```python
from build123d import *

# Parameters (mm, degrees)
SKETCH_1_W          = 95
SKETCH_1_H          = 45
EXTRUDE_1_DEPTH     = 19.3
SHELL_1_T           = -4
FILLET_1_R          = 4.5
SKETCH_2_W          = 71.05
SKETCH_2_H          = 22.55
CUT_EXTRUDE_1_DEPTH = 4.5
EXTRUDE_3_DEPTH     = 6
SKETCH_7_R          = 1.55
CUT_EXTRUDE_2_DEPTH = 4
SKETCH_8_R          = 0.75
EXTRUDE_5_DEPTH     = 5
EXTRUDE_6_DEPTH     = 2.5
SKETCH_9_W          = 1.5
SKETCH_9_H          = 22.55
EXTRUDE_7_DEPTH     = 2.5
SKETCH_10_W         = 74.05
SKETCH_10_H         = 26.962586992
CUT_EXTRUDE_3_DEPTH = 9
SKETCH_12_W         = 4.67
SKETCH_12_H         = 2.36
CUT_EXTRUDE_4_DEPTH = 24
FILLET_2_R          = 1
FILLET_3_R          = 1


with BuildPart() as part:
    # Sketch 1 → Extrude 1 (new body)
    with BuildSketch(Plane(origin=(0, 0, 0), x_dir=(1, 0, 0), z_dir=(0, 1, 0))):
        with Locations((47.5, -22.5)):
            Rectangle(SKETCH_1_W, SKETCH_1_H)
    extrude(amount=EXTRUDE_1_DEPTH)

    # Shell 1
    shell_1_openings = [part.faces().sort_by_distance(p)[0] for p in [
        (47.5, 19.3, 22.5),
    ]]
    offset(amount=SHELL_1_T, openings=shell_1_openings, kind=Kind.INTERSECTION)

    # Fillet 1
    fillet_1_edges = [part.edges().sort_by_distance(p)[0] for p in [
        (47.5, 0, 0),
        (95, 0, 22.5),
        (47.5, 0, 45),
        (0, 0, 22.5),
        (0, 9.65, 0),
        (95, 9.65, 0),
        (95, 9.65, 45),
        (0, 9.65, 45),
    ]]
    fillet(fillet_1_edges, radius=FILLET_1_R)

    # Sketch 2 → Cut-Extrude 1 (cut)
    with BuildSketch(Plane(origin=(0, 0, 0), x_dir=(-1, 0, 0), z_dir=(0, -1, 0))):
        with Locations((-47.5, -22.5)):
            Rectangle(SKETCH_2_W, SKETCH_2_H)
    extrude(amount=-CUT_EXTRUDE_1_DEPTH, mode=Mode.SUBTRACT)

    # Sketch 6 → Extrude 3 (add)
    with BuildSketch(Plane(origin=(0, 4, 0), x_dir=(1, 0, 0), z_dir=(0, 1, 0))):
        Polygon((11.975, -11.225), (11.975, -13.725), (7.475, -13.725), (7.475, -5.725), (15.475, -5.725), (15.475, -11.225), align=None)
        Polygon((11.975, -33.775), (11.975, -31.775), (7.475, -31.775), (7.475, -40.725), (15.475, -40.725), (15.475, -33.775), align=None)
        Polygon((87.525, -40.725), (79.525, -40.725), (79.525, -33.775), (83.025, -33.775), (83.025, -31.775), (87.525, -31.775), align=None)
        Polygon((79.525, -5.725), (79.525, -11.225), (83.025, -11.225), (83.025, -13.725), (87.525, -13.725), (87.525, -5.725), align=None)
    extrude(amount=EXTRUDE_3_DEPTH)

    # Sketch 7 → Cut-Extrude 2 (cut)
    with BuildSketch(Plane(origin=(0, 10, 0), x_dir=(1, 0, 0), z_dir=(0, 1, 0))):
        with Locations(Location((9.975, -7.725, 0), (0, 0, 270))):
            Circle(SKETCH_7_R)
        with Locations(Location((85.025, -7.725, 0), (0, 0, 90))):
            Circle(SKETCH_7_R)
        with Locations(Location((9.975, -38.725, 0), (0, 0, 270))):
            Circle(SKETCH_7_R)
        with Locations(Location((85.025, -38.725, 0), (0, 0, 90))):
            Circle(SKETCH_7_R)
    extrude(amount=-CUT_EXTRUDE_2_DEPTH, mode=Mode.SUBTRACT)

    # Sketch 8 → Extrude 5 (add)
    with BuildSketch(Plane(origin=(0, 19.3, 0), x_dir=(1, 0, 0), z_dir=(0, 1, 0))):
        with Locations((6, -43)):
            Circle(SKETCH_8_R)
        with Locations((6, -2)):
            Circle(SKETCH_8_R)
        with Locations((89, -2)):
            Circle(SKETCH_8_R)
        with BuildLine():
            ThreePointArc((89.75, -2), (89.530330086, -2.530330086), (89, -2.75))
            Line((89, -2.75), (92.25, -2.75))
            Line((92.25, -2.75), (92.25, -6))
            ThreePointArc((92.25, -6), (92.469669914, -5.469669914), (93, -5.25))
            Line((93, -5.25), (93, -2))
            Line((93, -2), (89.75, -2))
        make_face()
        with Locations((93, -6)):
            Circle(SKETCH_8_R)
        with Locations((93, -39)):
            Circle(SKETCH_8_R)
        with BuildLine():
            Line((92.25, -42.25), (89, -42.25))
            ThreePointArc((89, -42.25), (89.530330086, -42.469669914), (89.75, -43))
            Line((89.75, -43), (93, -43))
            Line((93, -43), (93, -39.75))
            ThreePointArc((93, -39.75), (92.469669914, -39.530330086), (92.25, -39))
            Line((92.25, -39), (92.25, -42.25))
        make_face()
        with Locations((89, -43)):
            Circle(SKETCH_8_R)
        with BuildLine():
            Line((6, -42.25), (2.75, -42.25))
            Line((2.75, -42.25), (2.75, -43))
            Line((2.75, -43), (5.25, -43))
            ThreePointArc((5.25, -43), (5.469669914, -42.469669914), (6, -42.25))
        make_face()
        with BuildLine():
            Line((5.25, -2), (2.75, -2))
            Line((2.75, -2), (2.75, -2.75))
            Line((2.75, -2.75), (6, -2.75))
            ThreePointArc((6, -2.75), (5.469669914, -2.530330086), (5.25, -2))
        make_face()
    extrude(amount=EXTRUDE_5_DEPTH)

    # Sketch 8_4 → Extrude 6 (add)
    with BuildSketch(Plane(origin=(0, 19.3, 0), x_dir=(1, 0, 0), z_dir=(0, 1, 0))):
        with BuildLine():
            ThreePointArc((6.75, -2), (6.530330086, -2.530330086), (6, -2.75))
            Line((6, -2.75), (89, -2.75))
            ThreePointArc((89, -2.75), (88.469669914, -2.530330086), (88.25, -2))
            Line((88.25, -2), (6.75, -2))
        make_face()
        with BuildLine():
            ThreePointArc((93, -6.75), (92.469669914, -6.530330086), (92.25, -6))
            Line((92.25, -6), (92.25, -39))
            ThreePointArc((92.25, -39), (92.469669914, -38.469669914), (93, -38.25))
            Line((93, -38.25), (93, -6.75))
        make_face()
        with BuildLine():
            Line((89, -42.25), (6, -42.25))
            ThreePointArc((6, -42.25), (6.530330086, -42.469669914), (6.75, -43))
            Line((6.75, -43), (88.25, -43))
            ThreePointArc((88.25, -43), (88.469669914, -42.469669914), (89, -42.25))
        make_face()
    extrude(amount=EXTRUDE_6_DEPTH)

    # Sketch 9 → Extrude 7 (add)
    with BuildSketch(Plane(origin=(0, 19.3, 0), x_dir=(1, 0, 0), z_dir=(0, 1, 0))):
        with Locations((2.75, -22.5)):
            Rectangle(SKETCH_9_W, SKETCH_9_H)
    extrude(amount=EXTRUDE_7_DEPTH)

    # Sketch 10 → Cut-Extrude 3 (cut)
    with BuildSketch(Plane(origin=(0, 10, 0), x_dir=(1, 0, 0), z_dir=(0, 1, 0))):
        with Locations((47.5, -23.243706504)):
            Rectangle(SKETCH_10_W, SKETCH_10_H)
    extrude(amount=-CUT_EXTRUDE_3_DEPTH, mode=Mode.SUBTRACT)

    # Sketch 12 → Cut-Extrude 4 (cut)
    with BuildSketch(Plane(origin=(95, 0, 0), x_dir=(0, 0, -1), z_dir=(1, 0, 0))):
        with Locations((-24.835, 18.12)):
            Rectangle(SKETCH_12_W, SKETCH_12_H)
        with Locations((-20.165, 18.12)):
            Rectangle(SKETCH_12_W, SKETCH_12_H)
        Polygon((-27.17, 19.3), (-22.5, 19.3), (-17.83, 19.3), (-17.83, 20.8), (-27.17, 20.8), align=None)
    extrude(amount=-CUT_EXTRUDE_4_DEPTH, mode=Mode.SUBTRACT)

    # Fillet 2
    fillet_2_edges = [part.edges().sort_by_distance(p)[0] for p in [
        (93, 16.94, 27.17),
    ]]
    fillet(fillet_2_edges, radius=FILLET_2_R)

    # Fillet 3
    fillet_3_edges = [part.edges().sort_by_distance(p)[0] for p in [
        (93, 16.94, 17.83),
    ]]
    fillet(fillet_3_edges, radius=FILLET_3_R)


solid = part.part
```
Check sheet for the modelled part. Datum: model origin and axes. Units: mm. A direction names the side the tool comes from. Round coordinates to 2 decimals unless told otherwise and drop trailing zeros. Loops run counter-clockwise (first coordinate to the right, second up) from the corner with the lowest first, then second, coordinate; pieces in that order, holes last. Notation, with made-up numbers: (-9.5, -17.75) - (26.5, -17.75) arc R31 ccw to (26.5, 15.25) - close; hole circle Ø9 at (11.5, -15.5). An arc over 180 degrees is marked (long way). Answer as a JSON object with one key per item and string values. Group by question number.
Q1. Sectioned sample at A-A, the plane z = 21.5. Enter the section's corners in (x, y) (3 decimals), plus the area to 3 significant figures.
Q2. Set-up check for faces 1 (the face through (91, 12, 23)), 2 (the face through (47, 12, 45)), 3 (the face through (4, 22, 43)): record each of +Z, -Z, +X, -X, +Y, -Y from which the full face is reachable in a straight line by a thin tool's end or side.
Q3. Sectioned sample at B-B, the plane x = 39. Enter the section's corners in (y, z) (3 decimals), plus the area to 3 significant figures.
Q4. Gauge pin test, flat ends, axial feed: P1, Ø4, axis at x = 85.025, z = 38.725, coming from the +Y side; P2, Ø1, axis at x = 91, y = 21, coming from the +Z side; P3, Ø2, axis at x = 59.5, z = 32, coming from the +Y side; P4, Ø4.5, axis at x = 93, z = 24, coming from the +Y side. Record the tip position at first contact, or that the pin passes through.
Q5. Mould release check, pull along X, two halves, no side actions. Record for faces 4 (the face through (47, 3.6, 9.762)), 5 (the face through (92.4, 24.3, 3.4)), 6 (the face through (93, 22, 4)): released by +X, released by -X, zero draft, split by the parting line, or undercut.
Q6. Scan lines: line 1 along X through (y, z) = (6.25, 9.5) (3 decimals); line 2 along Z through (x, y) = (68, 6); line 3 along X through (y, z) = (9.75, 19.5). Record each from-to range of solid material in increasing order. Write a range as [from, to].
Solution:
{
 "1": {"outline": "(0, 4.5) arc R4.5 ccw to (4.5, 0) - (11.975, 0) - (11.975, 1) - (10.475, 1) - (10.475, 4) - (4, 4) - (4, 19.3) - (3.5, 19.3) - (3.5, 21.8) - (2, 21.8) - (2, 19.3) - (0, 19.3) - close; (83.025, 0) - (90.5, 0) arc R4.5 ccw to (95, 4.5) - (95, 16.94) - (91, 16.94) - (91, 4) - (84.525, 4) - (84.525, 1) - (83.025, 1) - close; (92.25, 20.8) - (93, 20.8) - (93, 21.8) - (92.25, 21.8) - close", "area": "196 mm²"},
 "2": {"face 1": "+Y", "face 2": "+Z, +X, -X, +Y, -Y", "face 3": "+Z, -X, +Y"},
 "3": {"outline": "(0, 4.5) arc R4.5 ccw to (4.5, 0) - (19.3, 0) - (19.3, 2) - (21.8, 2) - (21.8, 2.75) - (19.3, 2.75) - (19.3, 4) - (4, 4) - (4, 9.762) - (1, 9.762) - (1, 11.225) - (0, 11.225) - close; (0, 33.775) - (1, 33.775) - (1, 36.725) - (4, 36.725) - (4, 41) - (19.3, 41) - (19.3, 42.25) - (21.8, 42.25) - (21.8, 43) - (19.3, 43) - (19.3, 45) - (4.5, 45) arc R4.5 ccw to (0, 40.5) - close", "area": "194 mm²"},
 "4": {"P1": "stops at y = 10", "P2": "stops at z = 43", "P3": "passes through", "P4": "stops at y = 21.8"},
 "5": {"face 4": "undercut", "face 5": "zero draft", "face 6": "released by +X"},
 "6": {"line 1": "x = [0, 4], [7.475, 15.475], [79.525, 87.525], [91, 95]", "line 2": "z = [0, 4], [41, 45]", "line 3": "x = [0, 4], [91, 95]"}
}
